Check sheet for the drawn part. Datum: minimum x, y, z corner. Units: mm. Round coordinates to 2 decimals unless told otherwise and drop trailing zeros.
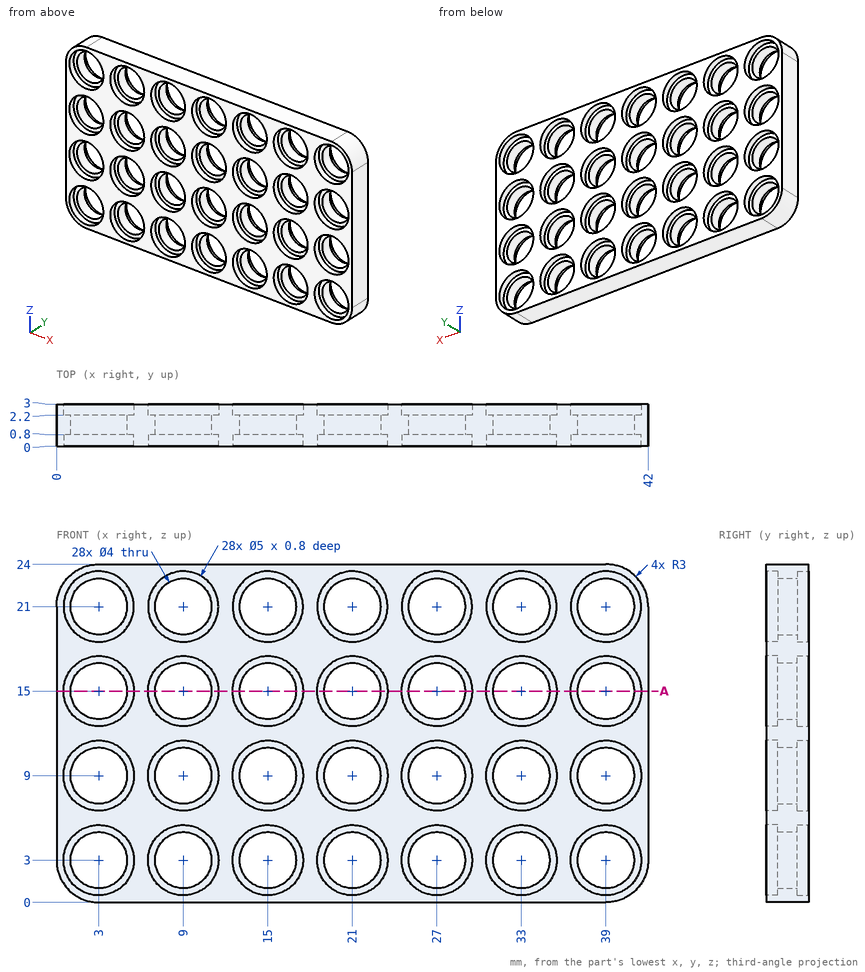
1) Sectioned sample at A-A on z = 15. Count the separate pieces of the cut face and the enclosed holes in it, and give its area (3 significant figures).
2) Gauge pin test, flat ends, axial feed: pin 1 (2.5 mm diameter, centred on x = 26, z = 14.5, fed in from +Y); pin 2 (4.5 mm diameter, centred on x = 3, z = 21, fed in from -Y). Record the tip position at first contact, or that the pin passes through.
3) Scan lines: line 1 (Z direction, x = 21, y = 0.4); line 2 (Z direction, x = 39, y = 1.45). Record each from-to range of solid material in increasing order.
Values found:
1. separate pieces: 8
1. enclosed holes: 0
1. area: 30.8 mm2
2. pin 1: stops at y = 2.2
2. pin 2: stops at y = 0.8
3. line 1: z = 0 to 0.5, 5.5 to 6.5, 11.5 to 12.5, 17.5 to 18.5, 23.5 to 24
3. line 2: z = 0 to 1, 5 to 7, 11 to 13, 17 to 19, 23 to 24
